from build123d import *

# Parameters (mm, degrees)
SKETCH1_W                    = 152
SKETCH1_H                    = 50
BASE_FLANGE1_DEPTH           = 8
EDGE_FLANGE1_STRIP_W         = 48
EDGE_FLANGE1_STRIP_H         = 8
EDGE_FLANGE1_STRIP_CUT_DEPTH = 152
EDGE_FLANGE1_DEPTH           = 152
CHAMFER1_SIZE                = 41
CHAMFER1_SIZE2               = 28.708509067
MIRROR3_START                = 53.078332384
MIRROR3_OUTLINE_W            = 53
MIRROR3_OUTLINE_H            = 14
MIRROR3_DEPTH                = 23.516633891


# Read off the part's stored shape, not the designer's step: Mirror3
# Sheet-metal steps are written as plain solids
with BuildPart() as part:
    # Sketch1 → Base-Flange1 (new body)
    with BuildSketch(Plane(origin=(0, 0, 0), x_dir=(1, 0, 0), z_dir=(0, 1, 0))):
        Rectangle(SKETCH1_W, SKETCH1_H)
    extrude(amount=-BASE_FLANGE1_DEPTH)

    # Edge-Flange1 strip (across the edge) → Edge-Flange1 strip cut (cut)
    with BuildSketch(Plane(origin=(-76, 0, 25), x_dir=(0, 0, -1), z_dir=(1, 0, 0))):
        with Locations((-8, -4)):
            Rectangle(EDGE_FLANGE1_STRIP_W, EDGE_FLANGE1_STRIP_H)
    extrude(amount=EDGE_FLANGE1_STRIP_CUT_DEPTH, mode=Mode.SUBTRACT)

    # Edge-Flange1 section (across the edge) → Edge-Flange1 (add)
    with BuildSketch(Plane(origin=(-76, 0, 25), x_dir=(0, 0, -1), z_dir=(1, 0, 0))):
        with BuildLine():
            Line((0, 8), (0, 32))
            Line((0, 32), (8, 32))
            Line((8, 32), (8, 8))
            ThreePointArc((8, 8), (10.343145751, 2.343145751), (16, 0))
            Line((16, 0), (16, -8))
            ThreePointArc((16, -8), (4.686291501, -3.313708499), (0, 8))
        make_face()
    extrude(amount=EDGE_FLANGE1_DEPTH)

    # Chamfer1
    chamfer1_edges = [part.edges().sort_by_distance(p)[0] for p in [
        (-76, -4, -25),
    ]]
    chamfer1_side = [part.faces().sort_by_distance(p)[0] for p in [
        (-76, -0.640312424, -8),
    ]]
    chamfer(chamfer1_edges, length=CHAMFER1_SIZE, length2=CHAMFER1_SIZE2, reference=chamfer1_side[0])

    # Mirror3 outline → Mirror3 (cut)
    with BuildSketch(Plane(origin=(0, 0, 0), x_dir=(0.5735764363510512, 0, 0.8191520442889882), z_dir=(0.8191520442889882, 0, -0.5735764363510512)).offset(MIRROR3_START)):
        with Locations((31.5, 1)):
            Rectangle(MIRROR3_OUTLINE_W, MIRROR3_OUTLINE_H)
    extrude(amount=MIRROR3_DEPTH, mode=Mode.SUBTRACT)


solid = part.part
Check sheet for the modelled part. Datum: model origin and axes. Units: mm. A direction names the side the tool comes from. Round coordinates to 2 decimals unless told otherwise and drop trailing zeros. Loops run counter-clockwise (first coordinate to the right, second up) from the corner with the lowest first, then second, coordinate; pieces in that order, holes last.
1. Sectioned sample at C-C on z = -20.5. Record the boundary of the cut face in (x, y).
2. Sectioned sample at A-A on x = -33. Record the boundary of the cut face in (y, z).
3. Sectioned sample at B-B on y = -4. Record the boundary of the cut face in (x, z), and give its area (3 significant figures).
4. Scan lines: probe 1 along Z at (x, y) = (-43, 11.5); probe 2 along Y at (x, z) = (-39, -12.5); probe 3 along Y at (x, z) = (-0.5, 15.5). Record each from-to range of solid material in increasing order.
5. Sectioned sample at D-D on x = 59.5. Record the boundary of the cut face in (y, z), and give its area (3 significant figures).
6. Set-up check for faces 1 (the flat face through (-1, 0, -8)), 2 (the flat face through (-1, 20, 25)): record each of +Z, -Z, +X, -X, +Y, -Y from which the full face is reachable in a straight line by a thin tool's end or side.
7. Gauge pin test, flat ends, axial feed: pin 1 Ø4 at (x, y) = (40, 15) entering from -Z; pin 2 Ø12 at (x, z) = (23.5, 4) entering from +Y; pin 3 Ø1.5 at (x, z) = (16, -3) entering from +Y. Record the tip position at first contact, or that the pin passes through.
Recorded:
1. outline: (-50.44, -8) - (50.44, -8) - (50.44, 0) - (-50.44, 0) - close
2. outline: (-8, -25) - (0, -25) - (0, 9) arc R8 cw to (8, 17) - (32, 17) - (32, 25) - (8, 25) arc R16 ccw to (-8, 9) - close
3. outline: (-76, 16) - (-47.29, -25) - (47.29, -25) - (76, 16) - (76, 19.58) - (-76, 19.58) - close
3. area: 5,600 mm2
4. probe 1: z = 17 to 25
4. probe 2: y = -8 to 0
4. probe 3: y = -6.62 to 3.34
5. outline: (-8, -7.56) - (0, -7.56) - (0, 9) arc R8 cw to (8, 17) - (32, 17) - (32, 25) - (8, 25) arc R16 ccw to (-8, 9) - close
5. area: 475 mm2
6. face 1: -Z, +X, -X, +Y
6. face 2: +Z, +X, -X, +Y, -Y
7. pin 1: stops at z = 17
7. pin 2: stops at y = 0.06
7. pin 3: stops at y = 0
